Source: three-view drawing plus pictorial views. Frame: mm from the lowest corner of the part. A direction names the side the tool comes from. Coordinates: 2 decimals unless noted, no trailing zeros. Loops run counter-clockwise (first coordinate to the right, second up) from the corner with the lowest first, then second, coordinate; pieces in that order, holes last. Notation, with made-up numbers: M 85,85.5 L 129,85.5 A16 ccw 129,109.5 Z; hole C -32,12.5 d4. An arc over 180 degrees is marked long. Use a Markdown table: item, result. Add a question column.
1. Section A-A on x = 44. Output: boundary loops of the cut face in (y, z), then the cut area to 3 significant figures.
2. Section C-C on y = 4. Output: boundary loops of the cut face in (x, z), then the cut area to 3 significant figures.
3. Line query: L1, parallel to Z at x = 52, y = 58.5; L2, parallel to X at y = 52, z = 148; L3, parallel to Y at x = 17, z = 191. Output: solid intervals per line, ascending. Write a range as [from, to].
4. Set-up query: the marked faces 1 and 2. Return all of +Z, -Z, +X, -X, +Y, -Y with unobstructed straight access to the full face (end or side cutting, diameter ignored); none if empty.
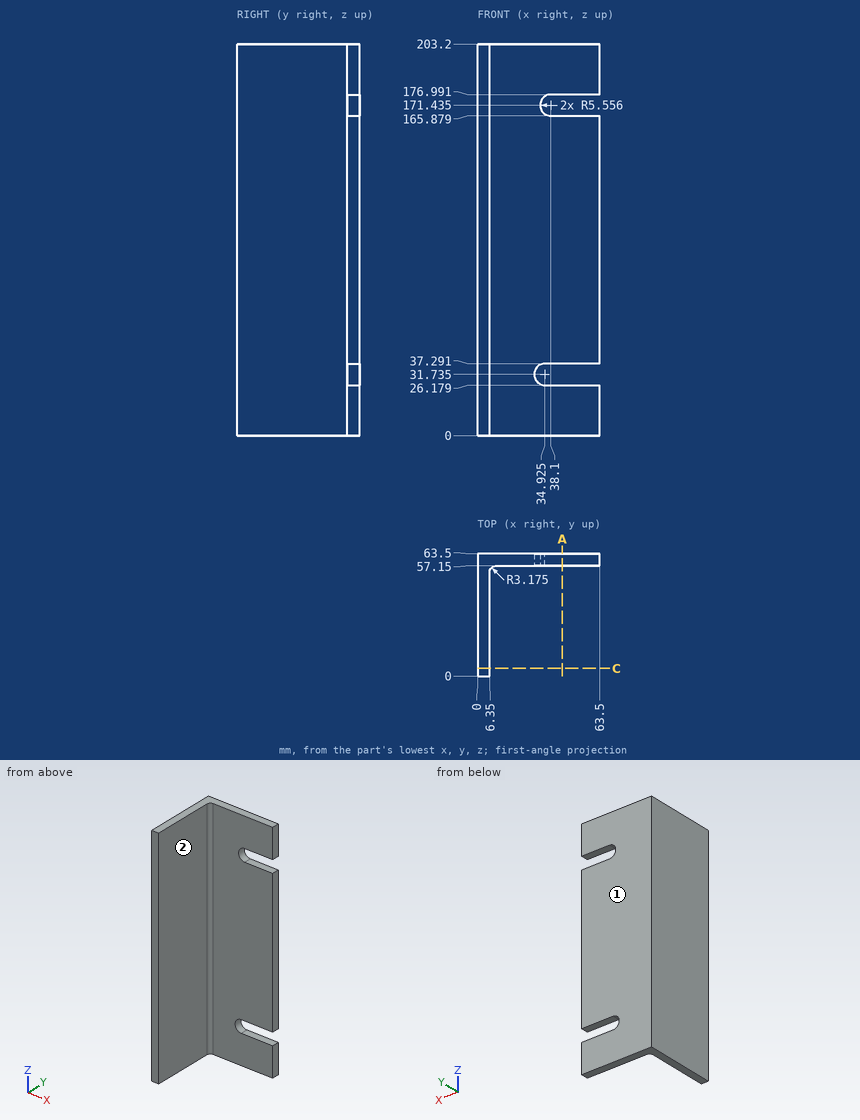
Answers below:
| question | item | result |
|---|---|---|
| 1 | outline | M 57.15,0 L 63.5,0 L 63.5,26.18 L 57.15,26.18 Z; M 57.15,37.29 L 63.5,37.29 L 63.5,165.88 L 57.15,165.88 Z; M 57.15,176.99 L 63.5,176.99 L 63.5,203.2 L 57.15,203.2 Z |
| 1 | area | 1,150 mm² |
| 2 | outline | M 0,0 L 6.35,0 L 6.35,203.2 L 0,203.2 Z |
| 2 | area | 1,290 mm² |
| 3 | L1 | z = [0, 26.18], [37.29, 165.88], [176.99, 203.2] |
| 3 | L2 | x = [0, 6.35] |
| 3 | L3 | y = [57.15, 63.5] |
| 4 | face 1 | +Z, -Z, +X, -X, +Y |
| 4 | face 2 | +Z, -Z, +X, -Y |
